Autodesk Inventor part; units mm, degrees
ref_plane "YZ Plane" through (0, 0, 0) normal (1, 0, 0) x (0, 1, 0)
ref_plane "XZ Plane" through (0, 0, 0) normal (0, 1, 0) x (-1, 0, 0)
ref_plane "XY Plane" through (0, 0, 0) normal (0, 0, 1) x (1, 0, 0)
sketch "Sketch1" plane through (0, 0, 0) normal (0, 1, 0) x (-1, 0, 0)
  line L0 (29, 0) -> (31, -2)
  line L1 (28, -35.353) -> (31, -32.353)
  line L2 (0, -32.353) -> (3, -35.353)
  line L3 (0, -2) -> (2, 0)
  line L4 (31, -2) -> (31, -32.353)
  line L5 (28, -35.353) -> (3, -35.353)
  line L6 (0, -32.353) -> (0, -2)
  line L7 (2, 0) -> (29, 0)
  point P0 (0, 0)
  dimension "d5" = 2
  dimension "d6" = 2
extrude "Extrusion1" add sketch "Sketch1" along normal blind 8
sketch "Sketch2" plane through (0, 0, -2) normal (1, 0, 0) x (0, 0, -1)
  line L0 (0, 0) -> (0, 8)
  line L1 (0, 8) -> (8.207, 8)
  line L2 (30.353, 8) -> (0, 8)
  line L3 (8.207, 8) -> (8.207, 5)
  circle A0 centre (8.207, 5) radius 1.6
  point P0 (-2, 0)
  dimension "d13" = 8.207
  dimension "d14" = 3
  dimension "d15" = 3.2
extrude "Extrusion2" cut sketch "Sketch2" against normal blind 31
sketch "Sketch3" plane through (0, 8, 0) normal (0, 1, 0) x (1, 0, 0)
  line L0 (-31, 2) -> (-29, 0)
  line L1 (-29, 0) -> (-39, 0)
  line L2 (-2, 0) -> (0, 2)
  line L3 (-2, 0) -> (8, 0)
  line L4 (-39, 0) -> (-39, 14.511)
  line L5 (8, 0) -> (8, 14.511)
  line L6 (8, 14.511) -> (-39, 14.511)
  line L7 (-29, 0) -> (-2, 0)
  point P0 (0, 0)
  dimension "d18" = 10
  dimension "d19" = 10
  dimension "d20" = 14.511
  dimension "d21" = 14.511
extrude "Extrusion3" add sketch "Sketch3" along normal blind 6
sketch "Sketch4" plane through (-29, 0, 0) normal (0, 0, 1) x (1, 0, 0)
  line L0 (-10, 14) -> (37, 14)
  line L1 (37, 14) -> (35, 14)
  line L2 (35, 14) -> (35, 12)
  circle A0 centre (35, 12) radius 2
  line L3 (-10, 8) -> (-10, 14)
  line L4 (-10, 14) -> (-8, 14)
  line L5 (-8, 14) -> (-8, 12)
  circle A1 centre (-8, 12) radius 2
  line L6 (-10, 14) -> (-10, 12)
  line L7 (37, 14) -> (37, 12)
  line L8 (37, 8) -> (37, 14)
  point P0 (29, 0)
  point P1 (-8, 14)
  dimension "d26" = 4
  dimension "d29" = 4
  dimension "d24" = 2
  dimension "d25" = 2
  dimension "d27" = 2
  dimension "d28" = 2
extrude "Extrusion4" cut sketch "Sketch4" against normal blind 14.511 contours L0 L7 A0 | L0 A1 L3
sketch "Sketch5" plane through (-29, 0, 0) normal (0, 0, 1) x (1, 0, 0)
  arc A0 (37, 12) -> (35, 14) centre (35, 12) ccw
  line L0 (35, 14) -> (30, 14)
  line L1 (35, 14) -> (-8, 14)
  line L2 (30, 14) -> (30, 11)
  line L3 (-8, 14) -> (-3, 14)
  line L4 (-3, 14) -> (-3, 11)
  circle A1 centre (-3, 11) radius 2
  circle A2 centre (30, 11) radius 2
  point P0 (29, 0)
  dimension "d32" = 5
  dimension "d33" = 3
  dimension "d34" = 5
  dimension "d35" = 3
  dimension "d36" = 4
  dimension "d37" = 4
extrude "Extrusion5" cut sketch "Sketch5" against normal blind 14.511
sketch "Sketch6" plane through (0, 8, 0) normal (0, 1, 0) x (1, 0, 0)
  line L0 (-28, 35.353) -> (-31, 32.353)
  line L1 (-28, 35.353) -> (-28, 24.409)
  line L2 (0, 32.353) -> (-3, 35.353)
  line L3 (-3, 35.353) -> (-3, 24.409)
  line L4 (-3, 24.409) -> (-28, 24.409)
  line L5 (-28, 35.353) -> (-3, 35.353)
  line L6 (-3, 35.353) -> (-28, 35.353)
  line L7 (-28, 35.353) -> (-15.5, 35.353)
  line L8 (-15.5, 35.353) -> (-15.5, 29.881)
  circle A0 centre (-15.5, 29.881) radius 2.5
  point P0 (0, 0)
  dimension "d40" = 10.944
  dimension "d41" = 10.944
  dimension "d42" = 12.5
  dimension "d43" = 5.472
  dimension "d44" = 5
extrude "Extrusion6" cut sketch "Sketch6" against normal blind 8 contours A0
sketch "Sketch7" plane through (8, 8, -14.511) normal (0, 0, -1) x (-1, 0, 0)
  line L0 (0, 0) -> (8, 0)
  line L1 (47, 0) -> (47, 4)
  line L2 (0, 0) -> (47, 0)
  line L3 (47, 0) -> (47, 6)
  line L4 (47, 6) -> (0, 6)
  line L5 (0, 6) -> (0, 0)
  point P0 (8, -8)
  dimension "d47" = 6
  dimension "d48" = 47
extrude "Extrusion7" cut sketch "Sketch7" against normal blind 7.2555
properties part number "camera_holder"
Model file for the job. Use its own axes, mm. A direction names the side the tool comes from. Give positions to 0.01 mm unless a question says otherwise; leave off trailing zeros. Write each loop counter-clockwise with the first axis right and the second up, starting at its lowest first coordinate (ties: lowest second). Pieces come first, ordered by that corner, then holes. Notation, with made-up numbers: M -4,78 L 46,78 A22 cw 46,84 Z; hole C -33.5,72.25 d8. An arc over 180 degrees is marked long. Use a Markdown table: item, result.
1) Pull direction Y, two halves, no side cores. Call faces 4 (the flat face through (-15, 0, -17)), 5 (the flat face through (-16, 14, -4)), 6 (the cylindrical face through (-30.092, 11.601, -3.577)), 7 (the flat face through (0, 4, -17)): +Y half, -Y half, draft (parallel to the pull), parting line (faces both ways), or undercut.
Responses:
| item | result |
|---|---|
| face 4 | -Y half |
| face 5 | +Y half |
| face 6 | undercut |
| face 7 | draft |
2) Tool access for faces 1 (the flat face through (-15, 11, -7.256)), 2 (the flat face through (-31, 4, -17)), 3 (the flat face through (-1, 4, -1)): list every direction of +Z, -Z, +X, -X, +Y, -Y with a clear straight run to the whole face (end or side of a thin tool).
Responses:
| item | result |
|---|---|
| face 1 | -Z, +X, -X, +Y |
| face 2 | +Z, -Z, -X, -Y |
| face 3 | +Z, +X, -Y |
3) Cut at B-B (x = -32). List the corners of the cut face in (y, z), and give its area (3 significant figures).
Responses:
| item | result |
|---|---|
| outline | M 8,-7.26 L 9,-7.26 L 9,0 L 8,0 Z; M 13,-7.26 L 14,-7.26 L 14,0 L 13,0 Z |
| area | 14.5 mm2 |
4) Drill centre lines: line 1 (X direction, y = 11, z = -1.25); line 2 (Z direction, x = -15.5, y = 6.25); line 3 (Z direction, x = -15.5, y = 4.5). Where is each one in solid material? Low to high. Write a range as from..to.
Responses:
| item | result |
|---|---|
| line 1 | x = -39..-34, -30..-1, 3..8 |
| line 2 | z = -35.35..-32.38, -27.38..-11.21, -9.21..0 |
| line 3 | z = -35.35..-32.38, -27.38..-11.73, -8.69..0 |
5) Cut at A-A (x = -15.5). List the corners of the cut face in (y, z), and give its area (3 significant figures).
Responses:
| item | result |
|---|---|
| outline | M 0,-35.35 L 8,-35.35 L 8,-32.38 L 0,-32.38 Z; M 0,-27.38 L 8,-27.38 L 8,-7.26 L 14,-7.26 L 14,0 L 0,0 Z; hole C 5,-10.21 d3.2 |
| area | 278 mm2 |
6) Pin check, flat tips, straight feed: pin 1 (2 mm diameter, centred on x = 4.5, z = -3.5, fed in from -Y); pin 2 (2.5 mm diameter, centred on y = 2.5, z = -23, fed in from +X); pin 3 (3 mm diameter, centred on x = -18, z = -25.5, fed in from +Y); pin 4 (2.5 mm diameter, centred on x = 1, y = 11, fed in from +Z). Stop position of each tip, or through.
Responses:
| item | result |
|---|---|
| pin 1 | stops at y = 8 |
| pin 2 | stops at x = 0 |
| pin 3 | stops at y = 8 |
| pin 4 | passes through |
7) Cut at D-D (x = -7). List the corners of the cut face in (y, z).
Responses:
| item | result |
|---|---|
| outline | M 0,-35.35 L 8,-35.35 L 8,-7.26 L 14,-7.26 L 14,0 L 0,0 Z; hole C 5,-10.21 d3.2 |
8) Cut at C-C (z = -4.5). List the corners of the cut face in (x, y), and give its area (3 significant figures).
Responses:
| item | result |
|---|---|
| outline | M -39,8 L -31,8 L -31,0 L 0,0 L 0,8 L 8,8 L 8,12 A2 ccw 6,14 L -37,14 A2 ccw -39,12 Z; hole C -32,11 d4; hole C 1,11 d4 |
| area | 503 mm2 |
